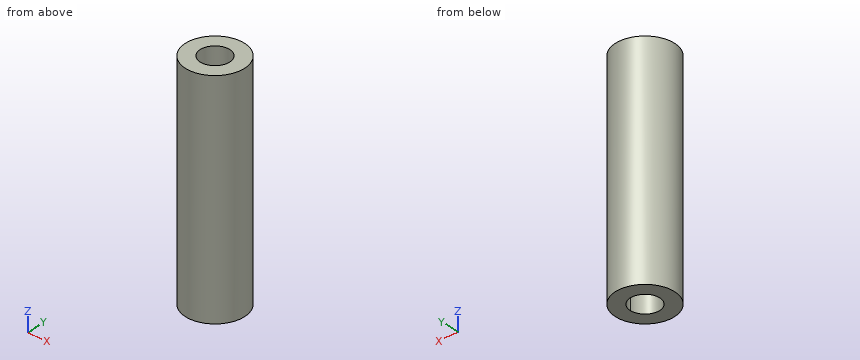
```python
from build123d import *

# Parameters (mm, degrees)
SKETCH_1_R               = 2.5
EXTRUDE_1_DEPTH          = 9.5
M3X0_5_1_D               = 2.5
M3X0_5_1_DEPTH           = 8.5
M3X0_5_1_TIP             = 0.751075774
M3X0_5_1_ON_FACE_2_D     = 2.5
M3X0_5_1_ON_FACE_2_DEPTH = 8.5
M3X0_5_1_ON_FACE_2_TIP   = 0.751075774
SKETCH_3_R               = 1.25
CUT_EXTRUDE_1_DEPTH      = 19


with BuildPart() as part:
    # ｽｹｯﾁ1 → ﾎﾞｽ - 押し出し1 (new body, symmetric)
    with BuildSketch(Plane.XY):
        Circle(SKETCH_1_R)
    extrude(amount=EXTRUDE_1_DEPTH, both=True)

    # M3x0.5 ねじ穴1
    with Locations(Plane.XY.offset(9.5)):
        with Locations((0, 0)):
            Hole(M3X0_5_1_D / 2, depth=M3X0_5_1_DEPTH)
            with Locations((0, 0, -(M3X0_5_1_DEPTH + M3X0_5_1_TIP / 2))):  # 118° drill point
                Cone(0, M3X0_5_1_D / 2, M3X0_5_1_TIP, mode=Mode.SUBTRACT)

    # M3x0.5 ねじ穴1 on face 2
    with Locations(Plane(origin=(0, 0, -9.5), x_dir=(-1, 0, 0), z_dir=(0, 0, -1))):
        with Locations((0, 0)):
            Hole(M3X0_5_1_ON_FACE_2_D / 2, depth=M3X0_5_1_ON_FACE_2_DEPTH)
            with Locations((0, 0, -(M3X0_5_1_ON_FACE_2_DEPTH + M3X0_5_1_ON_FACE_2_TIP / 2))):  # 118° drill point
                Cone(0, M3X0_5_1_ON_FACE_2_D / 2, M3X0_5_1_ON_FACE_2_TIP, mode=Mode.SUBTRACT)

    # ｽｹｯﾁ3 → ｶｯﾄ - 押し出し1 (cut)
    with BuildSketch(Plane(origin=(0, 0, -9.5), x_dir=(-1, 0, 0), z_dir=(0, 0, -1))):
        Circle(SKETCH_3_R)
    extrude(amount=-CUT_EXTRUDE_1_DEPTH, mode=Mode.SUBTRACT)


solid = part.part
```
The model under review builds one solid part; all positions refer to its coordinate system, in mm. Round coordinates to 2 decimals unless told otherwise and drop trailing zeros. Order: outer loops, then holes, each group sorted by start corner. A loop starts at its lowest first (then second) coordinate and runs counter-clockwise, first axis right, second up.
(1) Take a section at A-A, the plane x = 0. State the section outline as (y, z) points, plus the area to 3 significant figures.
Working result:
outline: (-2.5, -9.5) - (-1.25, -9.5) - (-1.25, 9.5) - (-2.5, 9.5) - close; (1.25, -9.5) - (2.5, -9.5) - (2.5, 9.5) - (1.25, 9.5) - close
area: 47.5 mm2
(2) Take a section at C-C, the plane y = 1.5. State the section outline as (x, z) points, plus the area to 3 significant figures.
Working result:
outline: (-2, -9.5) - (2, -9.5) - (2, 9.5) - (-2, 9.5) - close
area: 76.0 mm2
(3) Wall thickness on L1, parallel to X at y = 1.05, z = -8.5; L2, parallel to X at y = 0.8, z = -7; L3, parallel to Y at x = 0, z = 0: over which ranges is each line inside the solid? List them lowest first.
Working result:
L1: x = -2.27 to -0.68, 0.68 to 2.27
L2: x = -2.37 to -0.96, 0.96 to 2.37
L3: y = -2.5 to -1.25, 1.25 to 2.5
(4) Take a section at B-B, the plane z = -6.25. State the section outline as (x, y) points.
Working result:
outline: circle Ø5 at (0, 0); hole circle Ø2.5 at (0, 0)
(5) Take a section at D-D, the plane x = -2. State the section outline as (y, z) points.
Working result:
outline: (-1.5, -9.5) - (1.5, -9.5) - (1.5, 9.5) - (-1.5, 9.5) - close
